Check sheet for the modelled part. Datum: model origin and axes. Units: mm. A direction names the side the tool comes from. Coordinates: 2 decimals unless noted, no trailing zeros. Order: outer loops, then holes, each group sorted by start corner. A loop starts at its lowest first (then second) coordinate and runs counter-clockwise, first axis right, second up.
1. Cross-section at C-C (z = -3). Enter the section's corners in (x, y).
2. Cross-section at D-D (y = 5.75). Enter the section's corners in (x, z), then the cut area to 3 significant figures.
3. Cross-section at A-A (y = 2.25). Enter the section's corners in (x, z).
4. Gauge pin test, flat ends, axial feed: pin 1 Ø4 at (y, z) = (11.5, -10.5) entering from -X; pin 2 Ø3 at (x, z) = (7.5, -8.5) entering from -Y. Record the tip position at first contact, or that the pin passes through.
5. Thickness scan on line 1 (Z direction, x = 7.5, y = 7); line 2 (X direction, y = 6.25, z = -16); line 3 (Y direction, x = 1, z = -6.5). Record the ranges inside material, lowest first.
6. Set-up check for faces 1 (the flat face through (14.435, 10, -3)), 2 (the flat face through (-5.565, 10, -15)), 3 (the flat face through (-7.537, 5.607, -1.349)), 4 (the flat face through (5, 6, -13.295)): record each of +Z, -Z, +X, -X, +Y, -Y from which the full face is reachable in a straight line by a thin tool's end or side.
7. Cross-section at B-B (x = -5). Enter the section's corners in (y, z), then the cut area to 3 significant figures.
```python
from build123d import *

# Parameters (mm, degrees)
BOSS_EXTRUDE1_DEPTH = 12.5
BOSS_EXTRUDE4_DEPTH = 20
BOSS_EXTRUDE5_DEPTH = 4


with BuildPart() as part:
    # Sketch1 → Boss-Extrude1 (new body)
    with BuildSketch(Plane(origin=(0, 0, 0), x_dir=(1, 0, 0), z_dir=(0, 1, 0))):
        Polygon((-2.564516129, 3.29516129), (14.435483871, 3.29516129), (14.435483871, -2.70483871), (-5.564516129, -2.70483871), (-5.564516129, 3.29516129), (-4.064516129, 3.29516129), align=None)
    extrude(amount=BOSS_EXTRUDE1_DEPTH)

    # Sketch2 → Boss-Extrude4 (add)
    with BuildSketch(Plane(origin=(14.435483871, 0, 0), x_dir=(0, 0, -1), z_dir=(1, 0, 0))):
        Polygon((-2.70483871, 12.5), (13.29516129, 12.5), (13.29516129, 0), (17.29516129, 0), (17.29516129, 12.5), (17.29516129, 16.5), (-2.70483871, 16.5), align=None)
    extrude(amount=-BOSS_EXTRUDE4_DEPTH)

    # Sketch5 → Boss-Extrude5 (add)
    with BuildSketch(Plane.ZY.offset(5.564516129)):
        Polygon((-3.29516129, 0), (2.70483871, 0), (2.70483871, 16.5), (-3.29516129, 16.5), (-3.29516129, 11.338834765), (0.543673475, 7.5), (-3.29516129, 3.661165235), align=None)
    extrude(amount=BOSS_EXTRUDE5_DEPTH)


solid = part.part
```
Data:
1. outline: (-9.56, 0) - (14.44, 0) - (14.44, 16.5) - (-9.56, 16.5) - (-9.56, 11.04) - (-5.56, 11.04) - (-5.56, 3.96) - (-9.56, 3.96) - close
2. outline: (-9.56, -1.21) - (-5.56, -1.21) - (-5.56, -3.3) - (14.44, -3.3) - (14.44, 2.7) - (-9.56, 2.7) - close; (-5.56, -17.3) - (14.44, -17.3) - (14.44, -13.3) - (-5.56, -13.3) - close
2. area: 216 mm2
3. outline: (-9.56, -3.3) - (14.44, -3.3) - (14.44, 2.7) - (-9.56, 2.7) - close; (-5.56, -17.3) - (14.44, -17.3) - (14.44, -13.3) - (-5.56, -13.3) - close
4. pin 1: stops at x = -5.56
4. pin 2: stops at y = 12.5
5. line 1: z = -17.3 to -13.3, -3.3 to 2.7
5. line 2: x = -5.56 to 14.44
5. line 3: y = 12.5 to 16.5
6. face 1: +Z, -Z, +X, +Y, -Y
6. face 2: -Z, -X, +Y, -Y
6. face 3: -Z, -X
6. face 4: +X, -X, -Y
7. outline: (0, -17.3) - (16.5, -17.3) - (16.5, 2.7) - (0, 2.7) - (0, -3.3) - (12.5, -3.3) - (12.5, -13.3) - (0, -13.3) - close
7. area: 205 mm2
